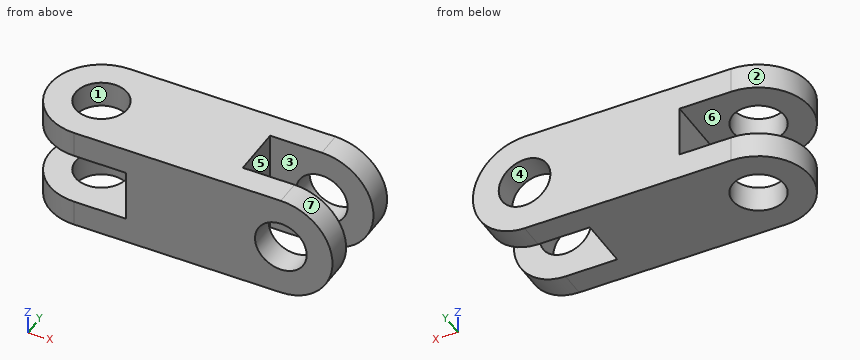
from build123d import *

# Parameters (mm, degrees)
ESQUISSE1_R        = 5
BOSS_EXTRU_1_DEPTH = 20
ESQUISSE2_R        = 5
BOSS_EXTRU_2_DEPTH = 20


with BuildPart() as part:
    # Esquisse1 → Boss.-Extru.1 (new body)
    with BuildSketch(Plane.XY):
        with BuildLine():
            Line((0, 0), (50, 0))
            Line((50, 0), (50, 5))
            Line((50, 5), (30, 5))
            Line((30, 5), (30, 15))
            Line((30, 15), (50, 15))
            Line((50, 15), (50, 20))
            Line((50, 20), (0, 20))
            ThreePointArc((0, 20), (-10, 10), (0, 0))
        make_face()
        with Locations((0, 10)):
            Circle(ESQUISSE1_R, mode=Mode.SUBTRACT)
    extrude(amount=BOSS_EXTRU_1_DEPTH)


with BuildPart() as body_2:
    # Esquisse2 → Boss.-Extru.2 (new body)
    with BuildSketch(Plane(origin=(0, 0, 0), x_dir=(1, 0, 0), z_dir=(0, 1, 0))):
        with BuildLine():
            Line((40, 0), (-10, 0))
            Line((-10, 0), (-10, -5))
            Line((-10, -5), (10, -5))
            Line((10, -5), (10, -15))
            Line((10, -15), (-10, -15))
            Line((-10, -15), (-10, -20))
            Line((-10, -20), (40, -20))
            ThreePointArc((40, -20), (50, -10), (40, 0))
        make_face()
        with Locations((40, -10)):
            Circle(ESQUISSE2_R, mode=Mode.SUBTRACT)
    extrude(amount=BOSS_EXTRU_2_DEPTH)

    # Combiner1: intersect part
    add(part.part, mode=Mode.INTERSECT)


solid = body_2.part
Here's how the part is built. I have some questions about the finished solid (model axes, mm). Face numbers are marked on the shaded views. A direction names the side the tool comes from. Coordinates: 2 decimals unless noted, no trailing zeros. Loops run counter-clockwise (first coordinate to the right, second up) from the corner with the lowest first, then second, coordinate; pieces in that order, holes last.
1. I need wall thicknesses on L1, parallel to Y at x = 0, z = 16.1; L2, parallel to X at y = 18.45, z = 10. Which ranges of each line are inside material? Lowest first, please.
2. If we mould it in two halves opening along Y, with no side actions, what happens to the marked faces 1, 2, 3 and 4? For each: pulls with the +Y half, pulls with the -Y half, needs draft (parallel to the pull), parting line crosses it, or undercut.
3. For P1, Ø6, axis at x = 38, z = 8, coming from the +Y side; P2, Ø4, axis at x = 39, z = 10.5, coming from the -Y side; P3, Ø11, axis at y = 12, z = 15, coming from the +X side; P4, Ø1, axis at y = 13, z = 10.5, coming from the +X side, each with a flat end and sliding along its axis, tell me the tip position at first contact or that it passes through.
4. Imagine slicing it at A-A, the plane z = 10. Please give me the cut outline in (x, y), and give its area (3 significant figures).
5. Imagine slicing it at C-C, the plane x = 44. Please give me the cut outline in (y, z).
6. Imagine slicing it at B-B, the plane y = 7. Please give me the cut outline in (x, z), and give its area (3 significant figures).
7. For the marked faces 5, 6 and 7, which set-ups out of +Z, -Z, +X, -X, +Y, -Y let a thin tool reach every point of the face, with its end or its side?
Taken from the geometry:
1. L1: y = 0 to 5, 15 to 20
1. L2: x = 10 to 35, 45 to 50
2. face 1: undercut
2. face 2: parting line crosses it
2. face 3: undercut
2. face 4: needs draft
3. P1: stops at y = 20
3. P2: passes through
3. P3: stops at x = 49.99
3. P4: stops at x = 30
4. outline: (10, 0) - (35, 0) - (35, 5) - (30, 5) - (30, 15) - (35, 15) - (35, 20) - (10, 20) - close; (45, 0) - (50, 0) - (50, 5) - (45, 5) - close; (45, 15) - (50, 15) - (50, 20) - (45, 20) - close
4. area: 500 mm2
5. outline: (0, 0.83) - (5, 0.83) - (5, 7) - (0, 7) - close; (0, 13) - (5, 13) - (5, 19.17) - (0, 19.17) - close; (15, 0.83) - (20, 0.83) - (20, 7) - (15, 7) - close; (15, 13) - (20, 13) - (20, 19.17) - (15, 19.17) - close
6. outline: (-9.54, 0) - (-4, 0) - (-4, 5) - (-9.54, 5) - close; (-9.54, 15) - (-4, 15) - (-4, 20) - (-9.54, 20) - close; (4, 0) - (30, 0) - (30, 20) - (4, 20) - (4, 15) - (10, 15) - (10, 5) - (4, 5) - close
6. area: 515 mm2
7. face 5: +Z, -Z, +X
7. face 6: -X, +Y, -Y
7. face 7: +X, +Y, -Y
